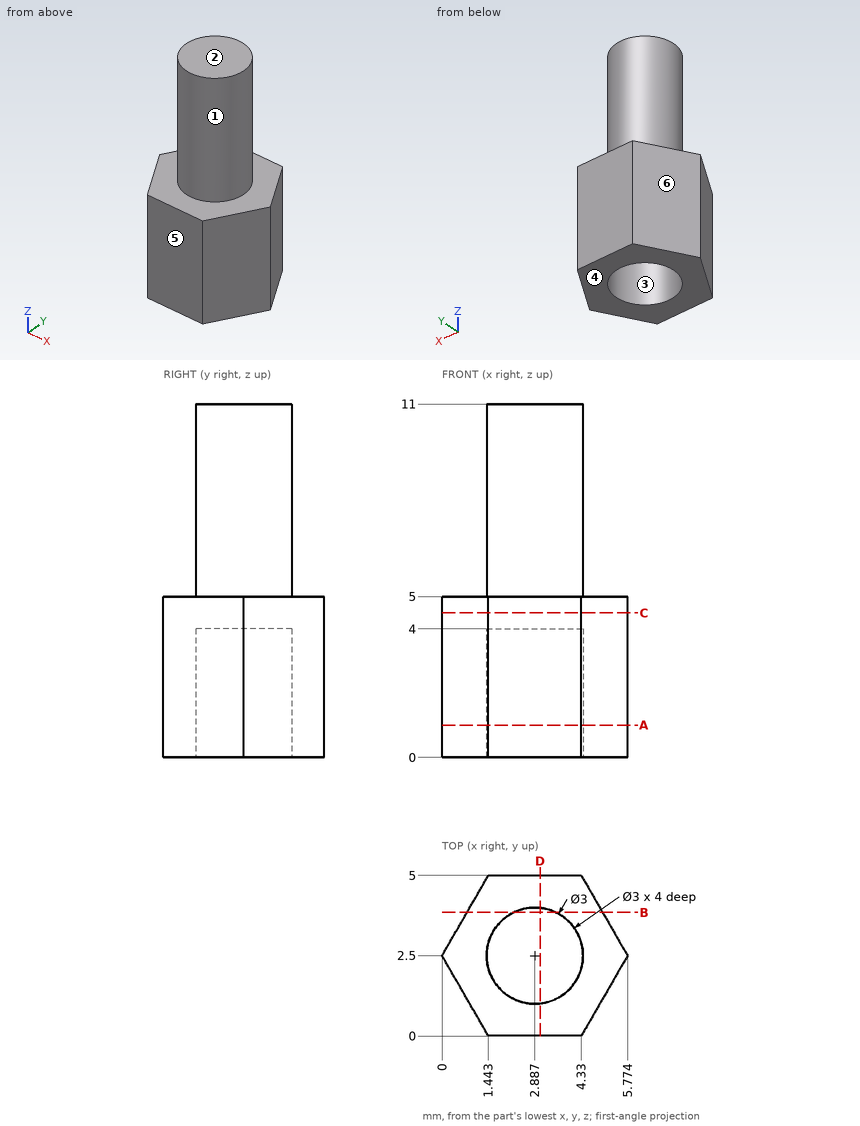
Drawing for the job (mm, zero at the part's lowest x, y, z). A direction names the side the tool comes from. Give positions to 0.01 mm unless a question says otherwise; leave off trailing zeros. Order: outer loops, then holes, each group sorted by start corner. A loop starts at its lowest first (then second) coordinate and runs counter-clockwise, first axis right, second up. Notation, with made-up numbers: M 24.5,53.5 L 29.5,53.5 A22 ccw 29.5,77.5 Z; hole C 39,-32.5 d9. An arc over 180 degrees is marked long. Use a Markdown table: item, result. Add a question column.
(1) Saw through at D-D, the plane x = 3.05. Give the cut face in (y, z).
(2) Drop flat-ended pins along their axis: P1, Ø1.5, axis at x = 4.5, z = 10, coming from the -Y side; P2, Ø2, axis at x = 1.5, z = 9, coming from the +Y side. Give the stop position or say it passes through.
(3) Saw through at C-C, the plane z = 4.5. Give the cut face in (x, y).
(4) Probe line 1 along Z through (x, y) = (0.65, 1.6); line 2 along Y through (x, z) = (3.7, 3); line 3 along Z through (x, y) = (3.6, 2.4). List the from-to ranges inside material, lowest first. Write a range as [from, to].
(5) Saw through at A-A, the plane z = 1. Give the cut face in (x, y), and give its area (3 significant figures).
(6) Saw through at B-B, the plane y = 3.85. Give the cut face in (x, z), and give its area (3 significant figures).
(7) Mould opens along Y. For the marked faces 3, 4, 5 and 6 say: +Y half, -Y half, draft (parallel to the pull), parting line (faces both ways), or undercut.
(8) 3-axis set-ups, long thin cutter, end or side, ignore diameter. For the marked faces 1 and 2: which of +Z, -Z, +X, -X, +Y, -Y reach the whole face in a straight line?
Answer key:
| question | item | result |
|---|---|---|
| 1 | outline | M 0,0 L 1.01,0 L 1.01,4 L 3.99,4 L 3.99,0 L 5,0 L 5,5 L 3.99,5 L 3.99,11 L 1.01,11 L 1.01,5 L 0,5 Z |
| 2 | P1 | y = 1.27 |
| 2 | P2 | y = 3.95 |
| 3 | outline | M 0,2.5 L 1.44,0 L 4.33,0 L 5.77,2.5 L 4.33,5 L 1.44,5 Z |
| 4 | line 1 | [0, 5] |
| 4 | line 2 | [0, 1.24], [3.76, 5] |
| 4 | line 3 | [4, 11] |
| 5 | outline | M 0,2.5 L 1.44,0 L 4.33,0 L 5.77,2.5 L 4.33,5 L 1.44,5 Z; hole C 2.89,2.5 d3 |
| 5 | area | 14.6 mm^2 |
| 6 | outline | M 0.78,0 L 2.23,0 L 2.23,4 L 3.54,4 L 3.54,0 L 4.99,0 L 4.99,5 L 3.54,5 L 3.54,11 L 2.23,11 L 2.23,5 L 0.78,5 Z |
| 6 | area | 23.7 mm^2 |
| 7 | face 3 | undercut |
| 7 | face 4 | draft |
| 7 | face 5 | -Y half |
| 7 | face 6 | +Y half |
| 8 | face 1 | +Z |
| 8 | face 2 | +Z, +X, -X, +Y, -Y |
